Here's how the part is built. I have some questions about the finished solid (model axes, mm). A direction names the side the tool comes from. Coordinates: 2 decimals unless noted, no trailing zeros. Answer as CSV lines item,"result". Start each with the question number.
Item 1: On a 3-axis mill with a long thin cutter (end or side, diameter ignored), from which of +Z, -Z, +X, -X, +Y, -Y can I reach the whole of each face in a straight line? I mean faces 1 (the face through (0, 0, 0)), 2 (the face through (-7.5, 3.175, 0.7)). Say none if no direction works.
Item 2: I need wall thicknesses on line 1 (Y direction, x = 7.5, z = 6.5) (3 decimals); line 2 (X direction, y = 0.5, z = -3); line 3 (Z direction, x = -6, y = 4.75). Which ranges of each line are inside material? Lowest first, please.
Item 3: I'm going to push flat-ended pins straight in: pin 1 (1.5 mm diameter, centred on x = 1, z = -0.5, fed in from -Y); pin 2 (1 mm diameter, centred on x = 3, y = 3, fed in from +Z); pin 3 (1.5 mm diameter, centred on x = -7, y = 2, fed in from +Z). Where does each tip first touch, or does it pass through?
from build123d import *

# Parameters (mm, degrees)
SKETCH2_W           = 19.05
SKETCH2_H           = 19.05
BOSS_EXTRUDE1_DEPTH = 3.175
BOSS_EXTRUDE1_TAPER = 8
SKETCH3_W           = 14.1575657
SKETCH3_H           = 14.1575657
BOSS_EXTRUDE2_DEPTH = 3.175
BOSS_EXTRUDE2_TAPER = 8


with BuildPart() as part:
    # Sketch2 → Boss-Extrude1 (new body)
    with BuildSketch(Plane(origin=(0, 0, 0), x_dir=(1, 0, 0), z_dir=(0, 1, 0))):
        Rectangle(SKETCH2_W, SKETCH2_H)
    extrude(amount=BOSS_EXTRUDE1_DEPTH, taper=BOSS_EXTRUDE1_TAPER)

    # Sketch3 → Boss-Extrude2 (add)
    with BuildSketch(Plane(origin=(0, 3.175, 0), x_dir=(1, 0, 0), z_dir=(0, 1, 0))):
        Rectangle(SKETCH3_W, SKETCH3_H)
    extrude(amount=BOSS_EXTRUDE2_DEPTH, taper=BOSS_EXTRUDE2_TAPER)


solid = part.part
Responses:
1,face 1,"+Z, -Z, +X, -X, -Y"
1,face 2,"+Y"
2,line 1,"y = 0 to 3.175"
2,line 2,"x = -9.45 to 9.45"
2,line 3,"z = -6.86 to 6.86"
3,pin 1,"stops at y = 0"
3,pin 2,"stops at z = 9.17"
3,pin 3,"stops at z = 9.35"
